Build history of the part. All positions in model axes, mm. A direction names the side the tool comes from. Give positions to 0.01 mm unless a question says otherwise; leave off trailing zeros. Answer in a Markdown table with one row per item. Add a question column.
```python
from build123d import *

# Parameters (mm, degrees)
F1_DEPTH = 25
F2_COUNT = 12
F3_R     = 40
F4_DEPTH = 10
F5_R     = 9.99999
F7_D     = 4


# Not quite as in the source:
# - a fillet or chamfer is up to 0.001 mm smaller than in the source, because OpenCascade refuses the exact size


with BuildPart() as f1:
    # F0 (on Top) → F1 (new body)
    with BuildSketch(Plane.XY):
        with BuildLine():
            ThreePointArc((-4.9937460889, 49.75), (-33.5433502766, -37.0788841825), (50, 0))
            ThreePointArc((50, 0), (37.0788841825, 33.5433502766), (4.9937460889, 49.75))
            ThreePointArc((4.9937460889, 49.75), (0, 45), (-4.9937460889, 49.75))
        make_face()
        with BuildLine():
            ThreePointArc((-4.9937460889, 49.75), (0, 45), (4.9937460889, 49.75))
            ThreePointArc((4.9937460889, 49.75), (0, 50), (-4.9937460889, 49.75))
        make_face()
        with BuildLine():
            ThreePointArc((-4.9937460889, 49.75), (0, 50), (4.9937460889, 49.75))
            ThreePointArc((4.9937460889, 49.75), (4.9984362777, 49.8749608947), (5, 50))
            ThreePointArc((5, 50), (-0.1250391053, 54.9984362777), (-4.9937460889, 49.75))
        make_face()
    extrude(amount=F1_DEPTH)

    # F2: F1 ×12 about axis
    f2_axis = Axis((0, 0, 0), (0, 0, -1))


with BuildPart() as f1_1:
    add(f1.part)
    for i in range(1, F2_COUNT):
        add(f1.part.rotate(f2_axis, i * 360 / F2_COUNT))

    # F3 (on face) → F4 (cut)
    with BuildSketch(Plane(origin=(0, 0, 0), x_dir=(1, 0, 0), z_dir=(0, 0, -1))):
        Circle(F3_R)
    extrude(amount=-F4_DEPTH, mode=Mode.SUBTRACT)

    # F5 (radius 10 in the source; OpenCascade refuses exactly that, so slightly less here)
    f5_edges = [f1_1.edges().sort_by_distance(p)[0] for p in [
        (-40, 0, 10),
    ]]
    fillet(f5_edges, radius=F5_R)

    # F7 (through all)
    with Locations(Plane.XY.offset(25)):
        with Locations((25, 43.3012701892), (43.3012701892, 25), (50, 0), (43.3012701892, -25), (25, -43.3012701892), (0, -50), (-25, -43.3012701892), (-43.3012701892, -25), (-50, 0), (-43.3012701892, 25), (-25, 43.3012701892), (0, 50)):
            Hole(F7_D / 2)


solid = f1_1.part
```
(1) Pin check, flat tips, straight feed: pin 1 (1 mm diameter, centred on x = 43, z = 5, fed in from -Y); pin 2 (3 mm diameter, centred on x = -42, z = 6.5, fed in from +Y); pin 3 (1 mm diameter, centred on y = 38.5, z = 12, fed in from +X). Stop position of each tip, or through.
(2) Wall check: line 1 (X direction, y = -43, z = 12.75); line 2 (Y direction, x = 0, z = 7.25); line 3 (Y direction, x = 25, z = 7). Give the ranges that are in metal, low to high.
(3) Slice it at A-A, the plane y = 0. State how many separate pieces and enclosed holes the cut face has, then the cut area to 3 significant figures.
(4) Pull direction Y, two halves, no side cores. Call faces 1 (the flat face through (-29, -28, 0)), 2 (the cylindrical face through (-12.832, 48.325, 12.325)), 3 (the cylindrical face through (-0.923, 48.226, 12.325)): +Y half, -Y half, draft (parallel to the pull), parting line (faces both ways), or undercut.
(5) Tool access for faces 4 (the cylindrical face through (-13.05, -48.267, 12.325)), 5 (the flat face through (0, 0, 10)), 6 (the cylindrical face through (48.325, 12.832, 12.325)), 7 (the cylindrical face through (13.05, 48.267, 12.325)), 8 (the cylindrical face through (-48.267, 13.05, 12.325)): list every direction of +Z, -Z, +X, -X, +Y, -Y with a clear straight run to the whole face (end or side of a thin tool).
Solution:
| question | item | result |
|---|---|---|
| 1 | pin 1 | y = -30 |
| 1 | pin 2 | y = 30 |
| 1 | pin 3 | x = 32.5 |
| 2 | line 1 | -29.99 to -26.98, -23.02 to 23.02, 26.98 to 29.99 |
| 2 | line 2 | -55 to -52, -48 to -36.89, 36.89 to 48, 52 to 55 |
| 2 | line 3 | -48.3 to -45.3, -41.3 to -27.47, 27.47 to 41.3, 45.3 to 48.3 |
| 3 | separate pieces | 3 |
| 3 | enclosed holes | 0 |
| 3 | area | 1,790 mm^2 |
| 4 | face 1 | draft |
| 4 | face 2 | +Y half |
| 4 | face 3 | undercut |
| 5 | face 4 | +Z, -Z, -Y |
| 5 | face 5 | -Z |
| 5 | face 6 | +Z, -Z, +X |
| 5 | face 7 | +Z, -Z, +Y |
| 5 | face 8 | +Z, -Z, -X |
